Can you work these out from the model? Positions are in its coordinate system, mm. Give positions to 0.01 mm unless a question says otherwise; leave off trailing zeros. One line per question, with ' | ' between items. Start each with the question number.
1) Please list where this line runs through material, in increasing order: line 1 along X through (y, z) = (2.75, 114.5). Write a range as [from, to].
2) If we section it at A-A, the plane x = -46.5: State how many separate pieces and enclosed holes the cut face has, plus the area to 3 significant figures.
3) I'm going to push a flat-ended pin straight in: pin 1 Ø2 at (x, z) = (-22, -10.5) entering from +Y. Where does the tip first touch, or does it pass through?
```python
from build123d import *

# Parameters (mm, degrees)
SKETCH1_W           = 127
SKETCH1_H           = 381
SKETCH1_W_2         = 114.3
SKETCH1_H_2         = 6.35
BOSS_EXTRUDE1_DEPTH = 4.365625


with BuildPart() as part:
    # Sketch1 → Boss-Extrude1 (new body)
    with BuildSketch(Plane(origin=(0, 0, 0), x_dir=(1, 0, 0), z_dir=(0, 1, 0))):
        Rectangle(SKETCH1_W, SKETCH1_H)
        with Locations((0, 161.925)):
            Rectangle(SKETCH1_W_2, SKETCH1_H_2, mode=Mode.SUBTRACT)
        with Locations((0, 174.625)):
            Rectangle(SKETCH1_W_2, SKETCH1_H_2, mode=Mode.SUBTRACT)
        with Locations((0, 149.225)):
            Rectangle(SKETCH1_W_2, SKETCH1_H_2, mode=Mode.SUBTRACT)
        with Locations((0, 136.525)):
            Rectangle(SKETCH1_W_2, SKETCH1_H_2, mode=Mode.SUBTRACT)
        with Locations((0, 123.825)):
            Rectangle(SKETCH1_W_2, SKETCH1_H_2, mode=Mode.SUBTRACT)
        with Locations((0, 111.125)):
            Rectangle(SKETCH1_W_2, SKETCH1_H_2, mode=Mode.SUBTRACT)
        with Locations((0, 98.425)):
            Rectangle(SKETCH1_W_2, SKETCH1_H_2, mode=Mode.SUBTRACT)
        with Locations((0, 85.725)):
            Rectangle(SKETCH1_W_2, SKETCH1_H_2, mode=Mode.SUBTRACT)
        with Locations((0, 73.025)):
            Rectangle(SKETCH1_W_2, SKETCH1_H_2, mode=Mode.SUBTRACT)
        with Locations((0, 60.325)):
            Rectangle(SKETCH1_W_2, SKETCH1_H_2, mode=Mode.SUBTRACT)
        with Locations((0, 47.625)):
            Rectangle(SKETCH1_W_2, SKETCH1_H_2, mode=Mode.SUBTRACT)
        with Locations((0, 34.925)):
            Rectangle(SKETCH1_W_2, SKETCH1_H_2, mode=Mode.SUBTRACT)
        with Locations((0, 22.225)):
            Rectangle(SKETCH1_W_2, SKETCH1_H_2, mode=Mode.SUBTRACT)
        with Locations((0, 9.525)):
            Rectangle(SKETCH1_W_2, SKETCH1_H_2, mode=Mode.SUBTRACT)
        with Locations((0, -3.175)):
            Rectangle(SKETCH1_W_2, SKETCH1_H_2, mode=Mode.SUBTRACT)
        with Locations((0, -15.875)):
            Rectangle(SKETCH1_W_2, SKETCH1_H_2, mode=Mode.SUBTRACT)
        with Locations((0, -28.575)):
            Rectangle(SKETCH1_W_2, SKETCH1_H_2, mode=Mode.SUBTRACT)
        with Locations((0, -41.275)):
            Rectangle(SKETCH1_W_2, SKETCH1_H_2, mode=Mode.SUBTRACT)
        with Locations((0, -53.975)):
            Rectangle(SKETCH1_W_2, SKETCH1_H_2, mode=Mode.SUBTRACT)
        with Locations((0, -66.675)):
            Rectangle(SKETCH1_W_2, SKETCH1_H_2, mode=Mode.SUBTRACT)
        with Locations((0, -79.375)):
            Rectangle(SKETCH1_W_2, SKETCH1_H_2, mode=Mode.SUBTRACT)
        with Locations((0, -92.075)):
            Rectangle(SKETCH1_W_2, SKETCH1_H_2, mode=Mode.SUBTRACT)
        with Locations((0, -104.775)):
            Rectangle(SKETCH1_W_2, SKETCH1_H_2, mode=Mode.SUBTRACT)
        with Locations((0, -117.475)):
            Rectangle(SKETCH1_W_2, SKETCH1_H_2, mode=Mode.SUBTRACT)
        with Locations((0, -130.175)):
            Rectangle(SKETCH1_W_2, SKETCH1_H_2, mode=Mode.SUBTRACT)
        with Locations((0, -142.875)):
            Rectangle(SKETCH1_W_2, SKETCH1_H_2, mode=Mode.SUBTRACT)
        with Locations((0, -155.575)):
            Rectangle(SKETCH1_W_2, SKETCH1_H_2, mode=Mode.SUBTRACT)
        with Locations((0, -168.275)):
            Rectangle(SKETCH1_W_2, SKETCH1_H_2, mode=Mode.SUBTRACT)
    extrude(amount=BOSS_EXTRUDE1_DEPTH)


solid = part.part
```
Results found:
1) line 1: x = [-63.5, -57.15], [57.15, 63.5]
2) separate pieces: 29 | enclosed holes: 0 | area: 887 mm²
3) pin 1: passes through
